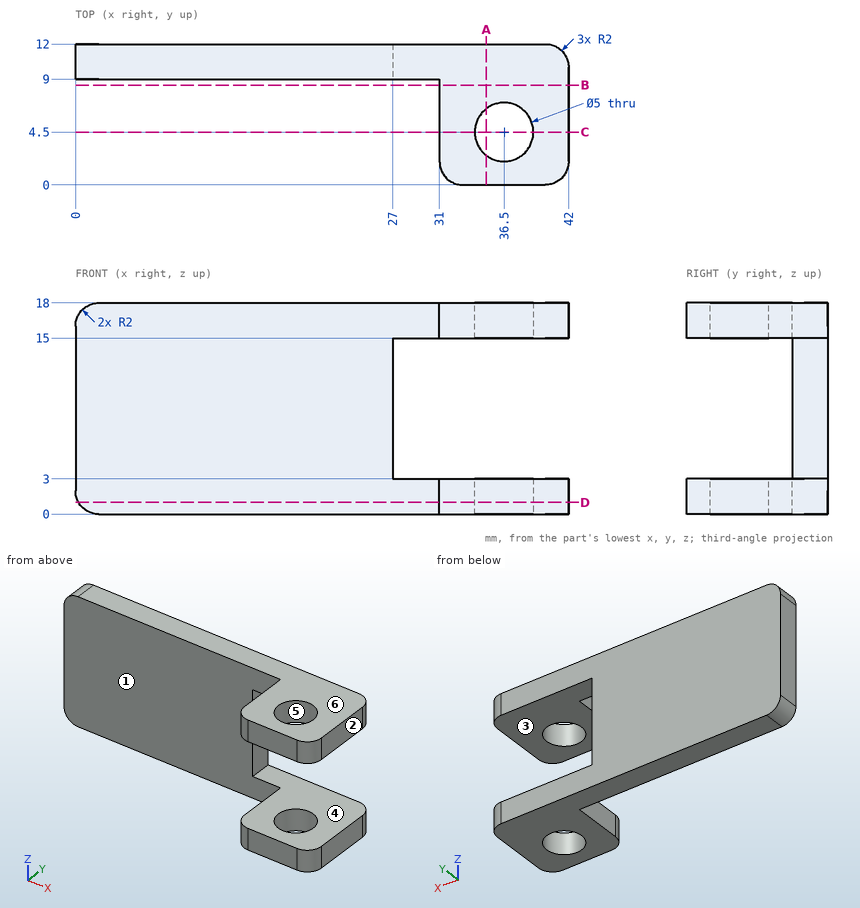
Study the drawing (mm; zero at the part's minimum x, y, z) and answer. A direction names the side the tool comes from. Coordinates: 2 decimals unless noted, no trailing zeros. Write each loop counter-clockwise with the first axis right and the second up, starting at its lowest first coordinate (ties: lowest second). Pieces come first, ordered by that corner, then holes. Notation, with made-up numbers: (-2.75, 66.5) - (49.25, 66.5) arc R23 ccw to (49.25, 86.5) - close; hole circle Ø3 at (-2.75, -17.5). An arc over 180 degrees is marked (long way). One line per question, with ' | ' between items.
1) Find section C-C, the plane y = 4.5. Determine the outline of the cut face in (x, z).
Checks:
outline: (31, 0) - (34, 0) - (34, 3) - (31, 3) - close; (31, 15) - (34, 15) - (34, 18) - (31, 18) - close; (39, 0) - (42, 0) - (42, 3) - (39, 3) - close; (39, 15) - (42, 15) - (42, 18) - (39, 18) - close
2) Find section D-D, the plane z = 1. Determine the outline of the cut face in (x, y).
Checks:
outline: (0.27, 9) - (31, 9) - (31, 2) arc R2 ccw to (33, 0) - (40, 0) arc R2 ccw to (42, 2) - (42, 10) arc R2 ccw to (40, 12) - (0.27, 12) - close; hole circle Ø5 at (36.5, 4.5)
3) Find section B-B, the plane y = 8.5. Determine the outline of the cut face in (x, z), and give its area (3 significant figures).
Checks:
outline: (31, 0) - (42, 0) - (42, 3) - (31, 3) - close; (31, 15) - (42, 15) - (42, 18) - (31, 18) - close | area: 66.0 mm2
4) Flat-ended cylindrical pins translate along their axes: P1, Ø0.9, axis at y = 11, z = 9.5, coming from the +X side; P2, Ø6, axis at x = 36.5, y = 4.5, coming from the +Z side; P3, Ø1, axis at x = 11.5, z = 9, coming from the -Y side; P4, Ø1.5, axis at y = 5, z = 16.5, coming from the -X side. Find the tip coordinate at first contact, or state that the pin passes through.
Checks:
P1: x = 27 | P2: z = 18 | P3: y = 9 | P4: x = 31
5) The mould has two halves that part along Z. Classify the marked faces 4, 5 and 6: +Z half, -Z half, draft (parallel to the pull), parting line (faces both ways), or undercut.
Checks:
face 4: undercut | face 5: draft | face 6: +Z half
6) For the marked faces 1, 2 and 3, determine the directions among +Z, -Z, +X, -X, +Y, -Y from which every point of the face is accessible in a straight line to the end or side of a thin tool.
Checks:
face 1: +Z, -Z, -X, -Y | face 2: +Z, -Z, +X, +Y, -Y | face 3: +X, +Y, -Y
7) Find section A-A, the plane x = 35. Determine the outline of the cut face in (y, z), and give its area (3 significant figures).
Checks:
outline: (0, 0) - (2.5, 0) - (2.5, 3) - (0, 3) - close; (0, 15) - (2.5, 15) - (2.5, 18) - (0, 18) - close; (6.5, 0) - (12, 0) - (12, 3) - (6.5, 3) - close; (6.5, 15) - (12, 15) - (12, 18) - (6.5, 18) - close | area: 48.0 mm2
8) Consider probe 1 along Y at (x, z) = (36.5, 0.95); probe 2 along Y at (x, z) = (11, 6.75); probe 3 along X at (y, z) = (7.75, 2.5). Determine where each line is inside the solid, lowest interval first. Write a range as [from, to].
Checks:
probe 1: [0, 2], [7, 12] | probe 2: [9, 12] | probe 3: [31, 42]
